from build123d import *

# Parameters (mm, degrees)
SKETCH1_W           = 25
SKETCH1_H           = 20
BOSS_EXTRUDE1_DEPTH = 3.175
SKETCH3_W           = 3.175
SKETCH3_H           = 20
BOSS_EXTRUDE2_DEPTH = 40
CHAMFER1_SIZE       = 0.5


with BuildPart() as part:
    # Sketch1 → Boss-Extrude1 (new body)
    with BuildSketch(Plane(origin=(0, 0, 0), x_dir=(1, 0, 0), z_dir=(0, 1, 0))):
        Rectangle(SKETCH1_W, SKETCH1_H)
    extrude(amount=BOSS_EXTRUDE1_DEPTH)

    # Sketch3 → Boss-Extrude2 (add)
    with BuildSketch(Plane(origin=(0, 3.175, 0), x_dir=(1, 0, 0), z_dir=(0, 1, 0))):
        with Locations((10.9125, 0)):
            Rectangle(SKETCH3_W, SKETCH3_H)
    extrude(amount=BOSS_EXTRUDE2_DEPTH)

    # Chamfer1
    chamfer1_edges = [part.edges().sort_by_distance(p)[0] for p in [
        (-12.5, 3.175, 0),
        (9.325, 3.175, 0),
        (12.5, 43.175, 0),
        (9.325, 43.175, 0),
        (-12.5, 0, 0),
        (12.5, 0, 0),
    ]]
    chamfer(chamfer1_edges, length=CHAMFER1_SIZE)


solid = part.part
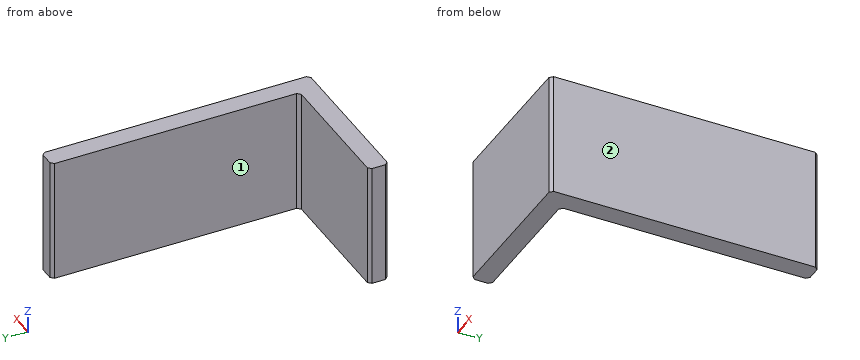
Build history of the part. All positions in model axes, mm. Face numbers are marked on the shaded views. A direction names the side the tool comes from. Coordinates: 2 decimals unless noted, no trailing zeros. Order: outer loops, then holes, each group sorted by start corner. A loop starts at its lowest first (then second) coordinate and runs counter-clockwise, first axis right, second up. Notation, with made-up numbers: (-9, 6) - (39, 6) arc R25 cw to (39, 30) - close; hole circle Ø6 at (13, 9.25). An arc over 180 degrees is marked (long way). Put each result on its own line as item: value.
1. Tool access for the marked faces 1 and 2: list every direction of +Z, -Z, +X, -X, +Y, -Y with a clear straight run to the whole face (end or side of a thin tool).
Answer sheet:
face 1: +Z, -Z, -X, +Y
face 2: +Z, -Z, +X, +Y, -Y
2. Drop flat-ended pins along their axis: P1, Ø10, axis at y = 34.5, z = 3.5, coming from the -X side (3 decimals); P2, Ø12, axis at x = -0.5, z = 3.5, coming from the +Y side (3 decimals). Give the stop position or say it passes through.
Answer sheet:
P1: stops at x = 9.325
P2: stops at y = 3.175
3. Saw through at C-C (y = 35). Write the cut outline in (x, z) (3 decimals).
Answer sheet:
outline: (9.325, -10) - (12.5, -10) - (12.5, 10) - (9.325, 10) - close
4. Probe line 1 along X through (y, z) = (29.5, -3) (3 decimals); line 2 along Y through (x, z) = (2.25, 2.5) (3 decimals); line 3 along X through (y, z) = (3, 3.5) (3 decimals). List the from-to ranges inside material, lowest first. Write a range as [from, to].
Answer sheet:
line 1: x = [9.325, 12.5]
line 2: y = [0, 3.175]
line 3: x = [-12.175, 12.5]
5. Saw through at B-B (x = -1.75). Write the cut outline in (y, z) (3 decimals), and give its area (3 significant figures).
Answer sheet:
outline: (0, -10) - (3.175, -10) - (3.175, 10) - (0, 10) - close
area: 63.5 mm^2
6. Saw through at A-A (z = -5.75). Write the cut outline in (x, y) (3 decimals).
Answer sheet:
outline: (-12.5, 0.5) - (-12, 0) - (12, 0) - (12.5, 0.5) - (12.5, 42.675) - (12, 43.175) - (9.825, 43.175) - (9.325, 42.675) - (9.325, 3.675) - (8.825, 3.175) - (-12, 3.175) - (-12.5, 2.675) - close
